from build123d import *

# Parameters (mm, degrees)
F0_W     = 109
F0_H     = 7
F0_R     = 3
F1_DEPTH = 3


# Not quite as in the source:
# - a feature names something its author has since deleted; it is built from what else it names


with BuildPart() as f1:
    # F0 (on Front) → F1 (new body)
    with BuildSketch(Plane.XZ):
        with BuildLine():
            Line((48.4662945779, -65), (53.4662945779, -65))
            Line((53.4662945779, -65), (53.4662945779, 0))
            Line((53.4662945779, 0), (20.9662945779, 22.9999753031))
            Line((20.9662945779, 22.9999753031), (-0.0337054221, 22.9999753031))
            Line((-0.0337054221, 22.9999753031), (0, 0))
            Line((0, 0), (-352, 0))
            Line((-352, 0), (-352, -39))
            Line((-352, -39), (-352, -55.5))
            Line((-352, -55.5), (-352, -80))
            ThreePointArc((-352, -80), (-349.9497474683, -84.9497474683), (-345, -87))
            Line((-345, -87), (-344, -87))
            ThreePointArc((-344, -87), (-339.0502525317, -84.9497474683), (-337, -80))
            Line((-337, -80), (-337, -70))
            Line((-337, -70), (-217, -70))
            Line((-217, -70), (-191, -72.5))
            ThreePointArc((-191, -72.5), (-188.1802970177, -61.3925278998), (-176.8015588718, -60.0320207981))
            Line((-176.8015588718, -60.0320207981), (-179, -72.5))
            Line((-179, -72.5), (-184.8187903634, -105.5))
            Line((-184.8187903634, -105.5), (-181.3187903634, -106))
            Line((-181.3187903634, -106), (-131.43, -111.007))
            Line((-131.43, -111.007), (-129.63038537, -100.8008782668))
            ThreePointArc((-129.63038537, -100.8008782668), (-126.3267144318, -96.2419842885), (-120.9729076822, -94.5))
            Line((-120.9729076822, -94.5), (-97.5, -94.5))
            Line((-97.5, -94.5), (-36.5, -94.5))
            Line((-36.5, -94.5), (3.4662945779, -182))
            Line((3.4662945779, -182), (-0.5337054221, -186.5))
            Line((-0.5337054221, -186.5), (1.4662945779, -189))
            Line((1.4662945779, -189), (8.4662945779, -190))
            Line((8.4662945779, -190), (44.4662945779, -169))
            Line((44.4662945779, -169), (45.4662945779, -166))
            Line((45.4662945779, -166), (47.9662945779, -164.5))
            Line((47.9662945779, -164.5), (12.9662945779, -104.5))
            ThreePointArc((12.9662945779, -104.5), (10.7409562508, -100.7720018727), (9.9662945779, -96.5))
            Line((9.9662945779, -96.5), (9.9662945779, -90.5))
            ThreePointArc((9.9662945779, -90.5), (10.599163398, -84.8597429137), (12.4662945779, -79.5))
            Line((12.4662945779, -79.5), (18.4662945779, -73.5))
            ThreePointArc((18.4662945779, -73.5), (22.6544664529, -70.6263437501), (27.4662945779, -69))
            Line((27.4662945779, -69), (48.4662945779, -65))
        make_face()
        with Locations((-266, -13)):
            Rectangle(F0_W, F0_H, mode=Mode.SUBTRACT)
        with Locations((-65, -69)):
            Circle(F0_R, mode=Mode.SUBTRACT)
    extrude(amount=F1_DEPTH)


solid = f1.part
Part model, mm, in its own coordinate system. A direction names the side the tool comes from. Coordinates: 2 decimals unless noted, no trailing zeros. Write each loop counter-clockwise with the first axis right and the second up, starting at its lowest first coordinate (ties: lowest second). Pieces come first, ordered by that corner, then holes. Notation, with made-up numbers: M 53.5,51 L 63.5,51 A14 cw 63.5,68 Z; hole C 80.25,-19.75 d4. An arc over 180 degrees is marked long. Return JSON: item names as keys, results as strings.
1. Probe L1, parallel to Z at x = -254, y = -0.9; L2, parallel to Z at x = -65, y = -1.35; L3, parallel to Z at x = -83.5, y = -1.3. List the from-to ranges inside material, lowest first.
Determined:
{"L1": "-70 to -16.5, -9.5 to 0", "L2": "-94.5 to -72, -66 to 0", "L3": "-94.5 to 0"}
2. Saw through at D-D, the plane x = -21. Write the cut outline in (y, z).
Determined:
{"outline": "M -3,-128.43 L 0,-128.43 L 0,0 L -3,0 Z"}
3. Saw through at A-A, the plane x = -310.5. Write the cut outline in (y, z), then the cut area to 3 significant figures.
Determined:
{"outline": "M -3,-70 L 0,-70 L 0,-16.5 L -3,-16.5 Z; M -3,-9.5 L 0,-9.5 L 0,0 L -3,0 Z", "area": "189 mm²"}
4. Saw through at B-B, the plane y = -1.3. Count the separate pieces of the cut face and the enclosed holes in it, then the cut area to 3 significant figures.
Determined:
{"separate pieces": "1", "enclosed holes": "2", "area": "38,100 mm²"}
5. Flat gauge pins, fed straight in: pin 1 Ø0.9 at (y, z) = (-1, -72.5) entering from +X; pin 2 Ø9.5 at (x, z) = (-65, -69) entering from -Y; pin 3 Ø0.9 at (x, y) = (-272, -1) entering from -Z; pin 4 Ø1.5 at (y, z) = (-2.5, -155.5) entering from +X. Where does each tip first touch, or does it go through?
Determined:
{"pin 1": "x = 20.27", "pin 2": "y = -3", "pin 3": "z = -70", "pin 4": "x = 43.15"}
6. Pull direction X, two halves, no side cores. Call faces 3 (the face through (-339.1, -1.5, -85)), 4 (the face through (-107, 0, -58)), 5 (the face through (-350, -1.5, -84.9)): pulls with the +X half, pulls with the -X half, needs draft (parallel to the pull), parting line crosses it, or undercut.
Determined:
{"face 3": "undercut", "face 4": "needs draft", "face 5": "pulls with the -X half"}
7. 3-axis set-ups, long thin cutter, end or side, ignore diameter. For faces 1 (the face through (30.7, -1.5, -134.9)), 2 (the face through (-107, -3, -58)): which of +Z, -Z, +X, -X, +Y, -Y reach the whole face in a straight line?
Determined:
{"face 1": "+X, +Y, -Y", "face 2": "+Z, -Z, +X, -X, -Y"}
8. Saw through at C-C, the plane x = -98. Write the cut outline in (y, z), then the cut area to 4 significant figures.
Determined:
{"outline": "M -3,-94.5 L 0,-94.5 L 0,0 L -3,0 Z", "area": "283.5 mm²"}
